```python
from build123d import *

# Parameters (mm, degrees)
SKETCH2_W                 = 96.2
SKETCH2_H                 = 40
SKETCH2_R                 = 1.5
SKETCH2_R_2               = 3.3734375
BOSS_EXTRUDE1_DEPTH       = 6
SKETCH3_R                 = 4.5
SKETCH3_R_2               = 1.5
BOSS_EXTRUDE2_DEPTH       = 4
MIRROR2_COPY_1_SKETCH_R   = 4.5
MIRROR2_COPY_1_SKETCH_R_2 = 1.5
MIRROR2_COPY_1_DEPTH      = 4
SKETCH5_R                 = 2.75
CUT_EXTRUDE1_DEPTH        = 3.3


with BuildPart() as part:
    # Sketch2 → Boss-Extrude1 (new body)
    with BuildSketch(Plane(origin=(0, 0, 0), x_dir=(1, 0, 0), z_dir=(0, 1, 0))):
        with Locations((70.631888672, 52.455394598)):
            Rectangle(SKETCH2_W, SKETCH2_H)
        with Locations((57.931888672, 39.755394598)):
            Circle(SKETCH2_R, mode=Mode.SUBTRACT)
        with Locations((83.331888672, 39.755394598)):
            Circle(SKETCH2_R, mode=Mode.SUBTRACT)
        with Locations((70.631888672, 52.455394598)):
            Circle(SKETCH2_R, mode=Mode.SUBTRACT)
        with Locations((57.931888672, 65.155394598)):
            Circle(SKETCH2_R, mode=Mode.SUBTRACT)
        with Locations((83.331888672, 65.155394598)):
            Circle(SKETCH2_R, mode=Mode.SUBTRACT)
        with Locations((108.731888672, 65.155394598)):
            Circle(SKETCH2_R_2, mode=Mode.SUBTRACT)
        with Locations((108.731888672, 39.755394598)):
            Circle(SKETCH2_R_2, mode=Mode.SUBTRACT)
        with Locations((32.531888672, 65.155394598)):
            Circle(SKETCH2_R_2, mode=Mode.SUBTRACT)
        with Locations((32.531888672, 39.755394598)):
            Circle(SKETCH2_R_2, mode=Mode.SUBTRACT)
    extrude(amount=BOSS_EXTRUDE1_DEPTH)

    # Sketch3 → Boss-Extrude2 (add)
    with BuildSketch(Plane(origin=(0, 6, 0), x_dir=(1, 0, 0), z_dir=(0, 1, 0))):
        with Locations((57.931888672, 65.155394598)):
            Circle(SKETCH3_R)
        with Locations((57.931888672, 65.155394598)):
            Circle(SKETCH3_R_2, mode=Mode.SUBTRACT)
    boss_extrude2 = extrude(amount=BOSS_EXTRUDE2_DEPTH)

    # Mirror1: Boss-Extrude2 across plane
    add(boss_extrude2.mirror(Plane.ZY.offset(-70.631888672)))

    # Mirror2: Boss-Extrude2 across plane
    add(boss_extrude2.mirror(Plane(origin=(0, 0, -52.455394598), x_dir=(1, 0, 0), z_dir=(0, 0, -1))))

    # Mirror2 copy 1 sketch → Mirror2 copy 1 (add)
    with BuildSketch(Plane(origin=(141.263777343, 6, -104.910789197), x_dir=(-1, 0, 0), z_dir=(0, 1, 0))):
        with Locations((57.931888672, 65.155394598)):
            Circle(MIRROR2_COPY_1_SKETCH_R)
        with Locations((57.931888672, 65.155394598)):
            Circle(MIRROR2_COPY_1_SKETCH_R_2, mode=Mode.SUBTRACT)
    extrude(amount=MIRROR2_COPY_1_DEPTH)

    # Sketch5 → Cut-Extrude1 (cut)
    with BuildSketch(Plane.XZ):
        with Locations((70.631888672, -52.455394598)):
            Circle(SKETCH5_R)
    extrude(amount=-CUT_EXTRUDE1_DEPTH, mode=Mode.SUBTRACT)


solid = part.part
```
Geometry check sheet. Reference: the model listing, model coordinates, mm. A direction names the side the tool comes from. Coordinates: 2 decimals unless noted, no trailing zeros. Order: outer loops, then holes, each group sorted by start corner. A loop starts at its lowest first (then second) coordinate and runs counter-clockwise, first axis right, second up.
Q1. Sectioned sample at A-A on x = 33. Record the cut outline in (y, z).
Reply:
outline: (0, -72.46) - (6, -72.46) - (6, -68.5) - (0, -68.5) - close; (0, -61.81) - (6, -61.81) - (6, -43.1) - (0, -43.1) - close; (0, -36.41) - (6, -36.41) - (6, -32.46) - (0, -32.46) - close
Q2. Sectioned sample at D-D on y = 1.75. Give the number of separate pieces and of enclosed holes in the cut face, and give its area (3 significant figures).
Reply:
separate pieces: 1
enclosed holes: 9
area: 3,650 mm2
Q3. Sectioned sample at C-C on x = 86. Record the cut outline in (y, z).
Reply:
outline: (0, -72.46) - (6, -72.46) - (6, -68.78) - (10, -68.78) - (10, -61.53) - (6, -61.53) - (6, -43.38) - (10, -43.38) - (10, -36.13) - (6, -36.13) - (6, -32.46) - (0, -32.46) - close
Q4. Thickness scan on probe 1 along Z at (x, y) = (33, 4); probe 2 along X at (y, z) = (2.5, -41); probe 3 along Y at (x, z) = (45.5, -67.5). Record the ranges inside material, lowest first.
Reply:
probe 1: z = -72.46 to -68.5, -61.81 to -43.1, -36.41 to -32.46
probe 2: x = 22.53 to 29.4, 35.67 to 57.09, 58.77 to 82.49, 84.17 to 105.6, 111.87 to 118.73
probe 3: y = 0 to 6
Q5. Draft check along Z on faces 1 (the face through (70, 3, -32.455)), 2 (the face through (105.36, 2.96, -65.3)), 3 (the face through (22.532, 3, -52)). Enter one of: released by +Z, released by -Z, zero draft, split by the parting line, or undercut.
Reply:
face 1: released by +Z
face 2: undercut
face 3: zero draft
Q6. Depth check by flat-ended pin: pin 1 Ø6 at (x, z) = (108.73, -65.16) entering from +Y; pin 2 Ø10 at (x, z) = (40, -68.5) entering from +Y; pin 3 Ø3 at (x, z) = (70, -52) entering from -Y. Enter the tip coordinate at first touch or a pass-through.
Reply:
pin 1: passes through
pin 2: stops at y = 6
pin 3: stops at y = 3.3
Q7. Tool access check on faces 4 (the face through (34.089, 2.958, -62.163)), 5 (the face through (67.885, 1.627, -52.334)), 6 (the face through (70, 6, -48)). Record the directions out of +Z, -Z, +X, -X, +Y, -Y that give a thin tool (end or side, any length) a straight path to the whole face; none if there is none.
Reply:
face 4: +Y, -Y
face 5: -Y
face 6: +Y
Q8. Sectioned sample at B-B on z = -47. Record the cut outline in (x, y).
Reply:
outline: (22.53, 0) - (118.73, 0) - (118.73, 6) - (22.53, 6) - close
